from build123d import *

# Parameters (mm, degrees)
F0_W     = 30.48
F0_H     = 101.6
F0_W_2   = 3.81
F1_DEPTH = 7.62
F2_DEPTH = 25.4
F4_DEPTH = 50.8


with BuildPart() as f1:
    # F0 (on Front) → F1 (new body)
    with BuildSketch(Plane.XZ):
        with Locations((-22.118616, 31.387416)):
            Rectangle(F0_W, F0_H)
        with Locations((-39.263616, 31.387416)):
            Rectangle(F0_W_2, F0_H)
        with Locations((-4.973616, 31.387416)):
            Rectangle(F0_W_2, F0_H)
    extrude(amount=F1_DEPTH)

    # F0 (on Front) → F2 (join)
    with BuildSketch(Plane.XZ):
        with Locations((-4.973616, 31.387416)):
            Rectangle(F0_W_2, F0_H)
        with Locations((-39.263616, 31.387416)):
            Rectangle(F0_W_2, F0_H)
    extrude(amount=-F2_DEPTH)

    # F3 (on face) → F4 (cut)
    with BuildSketch(Plane.YZ.offset(-3.068616)):
        Polygon((25.4, -19.412584), (25.4, -12.606675), (0, -19.412584), align=None)
    extrude(amount=-F4_DEPTH, mode=Mode.SUBTRACT)


solid = f1.part
Could you check a few things on this model? Use its own coordinates, in mm. A direction names the side the tool comes from. Coordinates: 2 decimals unless noted, no trailing zeros. Order: outer loops, then holes, each group sorted by start corner. A loop starts at its lowest first (then second) coordinate and runs counter-clockwise, first axis right, second up.
Q1. Suppose I cut it at C-C on x = -20. Please give me the cut outline in (y, z), and give its area (3 significant figures).
Q2. Which directions (+Z, -Z, +X, -X, +Y, -Y) give clear straight access to the entire face, cutting with the end or side of a thin tool? Please do faces 1 (the flat face through (-22, -2, 82.187)), 2 (the flat face through (-37.359, 13, 31)).
Q3. Will these pins go through, and if not, where does the flat tip stop? pin 1 (1 mm diameter, centred on x = -30.5, z = 46, fed in from +Y); pin 2 (12 mm diameter, centred on x = -14.5, y = 18, fed in from -Z).
Q4. Please list where these lines run through material, in increasing order: L1, parallel to X at y = 19.5, z = -2; L2, parallel to Y at x = -15, z = 59; L3, parallel to Z at x = -38, y = 22.
Q5. Suppose I cut it at B-B on z = 47.5. Please give me the cut outline in (x, y).
Q6. Thinking about a two-plate mould opening in X: for faces 3 (the flat face through (-41.169, 9, 31)), 4 (the flat face through (-22, 0, 32)), 5 (the flat face through (-4.95, 12.88, -15.96)), which applies, released by +X, released by -X, zero draft, split by the parting line, or undercut?
Q7. Suppose I cut it at A-A on y = 14. Please give me the cut outline in (x, z), and give its area (3 significant figures).
Q8. Suppose I cut it at D-D on y = 2.5. Please give me the cut outline in (x, z).
Answer:
1. outline: (-7.62, -19.41) - (0, -19.41) - (0, 82.19) - (-7.62, 82.19) - close
1. area: 774 mm2
2. face 1: +Z, +X, -X, +Y, -Y
2. face 2: +Z, -Z, +Y
3. pin 1: stops at y = 0
3. pin 2: passes through
4. L1: x = -41.17 to -37.36, -6.88 to -3.07
4. L2: y = -7.62 to 0
4. L3: z = -13.52 to 82.19
5. outline: (-41.17, -7.62) - (-3.07, -7.62) - (-3.07, 25.4) - (-6.88, 25.4) - (-6.88, 0) - (-37.36, 0) - (-37.36, 25.4) - (-41.17, 25.4) - close
6. face 3: released by -X
6. face 4: undercut
6. face 5: zero draft
7. outline: (-41.17, -15.66) - (-37.36, -15.66) - (-37.36, 82.19) - (-41.17, 82.19) - close; (-6.88, -15.66) - (-3.07, -15.66) - (-3.07, 82.19) - (-6.88, 82.19) - close
7. area: 746 mm2
8. outline: (-41.17, -18.74) - (-37.36, -18.74) - (-37.36, 82.19) - (-41.17, 82.19) - close; (-6.88, -18.74) - (-3.07, -18.74) - (-3.07, 82.19) - (-6.88, 82.19) - close
